Design review of the part built by this model. Coordinates are the model's own, in mm. A direction names the side the tool comes from. Give positions to 0.01 mm unless a question says otherwise; leave off trailing zeros. Write each loop counter-clockwise with the first axis right and the second up, starting at its lowest first coordinate (ties: lowest second). Pieces come first, ordered by that corner, then holes. Notation, with made-up numbers: (89.5, 10) - (100.5, 10) arc R23 ccw to (100.5, 23) - close; hole circle Ø9 at (72, -33). An arc over 180 degrees is marked (long way). Write each question's results on one line, items separated by ' | '. Start each with the question number.
Autodesk Inventor part; units mm, degrees
ref_plane "YZ Plane" through (0, 0, 0) normal (1, 0, 0) x (0, 1, 0)
ref_plane "XZ Plane" through (0, 0, 0) normal (0, 1, 0) x (-1, 0, 0)
ref_plane "XY Plane" through (0, 0, 0) normal (0, 0, 1) x (1, 0, 0)
sketch "Sketch1" plane through (0, 0, 0) normal (0, 1, 0) x (-1, 0, 0)
  circle A0 centre (0, 0) radius 33.655
  circle A1 centre (0, 0) radius 30.48
  dimension "d0" = 67.31
  dimension "d1" = 60.96
extrude "Extrusion1" add sketch "Sketch1" along normal blind 12.7
sketch "Sketch2" plane through (0, 12.7, 0) normal (0, 1, 0) x (1, 0, 0)
  circle A0 centre (0, 0) radius 33.655
extrude "Extrusion2" add sketch "Sketch2" along normal blind 9.525
sketch "Sketch3" plane through (0, 22.225, 0) normal (0, 1, 0) x (1, 0, 0)
  line L0 (18.0975, -25.7175) -> (-18.0975, -25.7175)
  line L1 (-18.0975, -25.7175) -> (-18.0975, 25.7175)
  line L2 (-18.0975, 25.7175) -> (18.0975, 25.7175)
  line L3 (18.0975, 25.7175) -> (18.0975, -25.7175)
  line L4 (18.0975, -25.7175) -> (-18.0975, 25.7175) construction
  line L5 (-18.0975, -25.7175) -> (18.0975, 25.7175) construction
  point P0 (0, 0)
  dimension "d6" = 36.195
  dimension "d7" = 51.435
extrude "Extrusion3" cut sketch "Sketch3" against normal blind 3.175
sketch "Sketch4" plane through (0, 19.05, 0) normal (0, 1, 0) x (1, 0, 0)
  line L0 (15.24, -22.86) -> (-15.24, -22.86)
  line L1 (-15.24, -22.86) -> (-15.24, 22.86)
  line L2 (-15.24, 22.86) -> (15.24, 22.86)
  line L3 (15.24, 22.86) -> (15.24, -22.86)
  line L4 (15.24, -22.86) -> (-15.24, 22.86) construction
  line L5 (-15.24, -22.86) -> (15.24, 22.86) construction
  point P0 (0, 0)
  dimension "d10" = 30.48
  dimension "d11" = 45.72
extrude "Extrusion4" cut sketch "Sketch4" against normal through all
ref_plane "Work Plane1" through (0, 6.35, 0) normal (0, -1, 0) x (1, 0, 0)
sketch "Sketch5" plane through (0, 6.35, 0) normal (0, -1, 0) x (1, 0, 0)
  circle A0 centre (0, 0) radius 33.655
  circle A1 centre (0, 0) radius 29.8345
  circle A2 centre (0, 0) radius 39.6875
  dimension "d15" = 79.375
extrude "Extrusion5" add sketch "Sketch5" against normal blind 3.175 contours A2
properties part number "Upper Coll r2ar"
Q1. For line 1 along Z through (x, y) = (0, 8); line 2 along Z through (x, y) = (0, 6.25) (3 decimals); line 3 along Y through (x, z) = (-23, 2.5) (3 decimals), list the stretches that pass through material, from the lowest coordinate up. Write a range as [from, to].
Q2. The part is to be moulded in two halves that separate along X. For faces 1 (the face through (-18, 9.525, -29)), 2 (the face through (7.296, 15.786, 32.855)), 3 (the face through (0, 16, -22.86)), say which applies: +X half, -X half, draft (parallel to the pull), parting line (faces both ways), or undercut.
Q3. Add section D-D on y = 8.5. State the section outline as (x, z) points (1 decimal), plus the area to 3 significant figures.
Q4. Insertion check: P1, Ø1, axis at x = -10, y = 8.5, coming from the -Z side; P2, Ø7, axis at y = 17, z = -4.5, coming from the +X side; P3, Ø1.6, axis at y = 20, z = -10, coming from the -X side. Each pin has a flat end and moves straight along its axis. Give the tip position at first contact, or say it passes through.
Q5. Add section C-C on y = 14.75. State the section outline as (x, z) points (3 decimals).
Q6. Machinability: for faces 4 (the face through (7.296, 3.131, 32.855)), 5 (the face through (18.098, 21, 0)), 6 (the face through (-15.24, 16, 0)), 7 (the face through (18, 0, 25)), which of the approach directions +Z, -Z, +X, -X, +Y, -Y give a long, thin tool a straight path to every point of the face, cutting with its end or side? Answer none if there is none.
Result:
1) line 1: z = [-39.69, -30.48], [30.48, 39.69] | line 2: z = [-33.655, -30.48], [30.48, 33.655] | line 3: y = [12.7, 22.225]
2) face 1: draft | face 2: parting line | face 3: undercut
3) outline: circle Ø79.4 at (0, 0); hole circle Ø61 at (0, 0) | area: 2,030 mm²
4) P1: stops at z = -38.53 | P2: stops at x = 33.64 | P3: stops at x = -32.37
5) outline: circle Ø67.31 at (0, 0); hole (-15.24, -22.86) - (15.24, -22.86) - (15.24, 22.86) - (-15.24, 22.86) - close
6) face 4: -Y | face 5: +Y | face 6: +Y, -Y | face 7: +Z, -Z, +X, -X, -Y
